Geometry: final body of the model. Coordinates: model frame, mm. A direction names the side the tool comes from. Give positions to 0.01 mm unless a question says otherwise; leave off trailing zeros. Order: outer loops, then holes, each group sorted by start corner. A loop starts at its lowest first (then second) coordinate and runs counter-clockwise, first axis right, second up. Notation, with made-up numbers: (22, -29.5) - (72, -29.5) arc R20 cw to (72, -16.5) - close; hole circle Ø9 at (30, -19). An arc over 180 degrees is marked (long way). Write item = value, one per line. Start each with the question number.
from build123d import *

# Parameters (mm, degrees)
FILLET1_R = 0.5


with BuildPart() as part:
    # Sketch1 → Revolve1 (revolve)
    with BuildSketch(Plane.XY, mode=Mode.PRIVATE) as revolve1_sk:
        Polygon((-80.816688046, 15.015), (-37.316688046, 15.015), (-24.316688046, 15.015), (-24.316688046, 17.5), (27.280476237, 17.5), (54.816688046, 17.5), (54.816688046, 22.5), (59.816688046, 22.5), (59.816688046, 17.5175), (80.816688046, 17.5175), (80.816688046, 0), (-80.816688046, 0), align=None)
    revolve(revolve1_sk.sketch.rotate(Axis((-91.454349808, 0, 0), (1, 0, 0)), 180), axis=Axis((-91.454349808, 0, 0), (1, 0, 0)))

    # Fillet1
    fillet1_edges = [part.edges().sort_by_distance(p)[0] for p in [
        (-24.316688046, 15.015, 0),
        (54.816688046, 17.5, 0),
        (59.816688046, 17.5175, 0),
    ]]
    fillet(fillet1_edges, radius=FILLET1_R)


solid = part.part
Q1. Contact query for flat-ended pins moving along their axis: pin 1 (1 mm diameter, centred on x = 38.5, y = 7.5, fed in from +Z); pin 2 (1.5 mm diameter, centred on x = 10.5, z = -4, fed in from -Y); pin 3 (12 mm diameter, centred on x = -9.5, z = 17.5, fed in from -Y). Output: stop coordinate, or through.
Q2. Section A-A, the plane y = 0. Return the cut outline in (x, z) (1 decimal).
Q3. Material intervals for line 1 along Y through (x, z) = (25, -9); line 2 along Z through (x, y) = (-10.5, 1); line 3 along X through (y, z) = (7, -16.5), sorted ascending. Write a range as from..to.
Q4. Section D-D, the plane x = -14.5. Return the cut outline in (y, z).
Q5. Section C-C, the plane x = -63. Return the cut outline in (y, z) (3 decimals), then the cut area to 3 significant figures.
Q6. Set-up query: faces 1 (the cylindrical face through (57.352, -10.382, 19.961)), 2 (the cylindrical face through (70.71, -16.71, -5.26)), 3 (the flat face through (54.817, -10.1, -15.1)). Return all of +Z, -Z, +X, -X, +Y, -Y with unobstructed straight access to the full face (end or side cutting, diameter ignored); none if empty.
The answers:
q1.pin_1 = 16.04
q1.pin_2 = -17.2
q1.pin_3 = -13.19
q2.outline = (-80.8, -15) - (-24.8, -15) arc R0.5 cw to (-24.3, -15.5) - (-24.3, -17.5) - (54.3, -17.5) arc R0.5 cw to (54.8, -18) - (54.8, -22.5) - (59.8, -22.5) - (59.8, -18) arc R0.5 cw to (60.3, -17.5) - (80.8, -17.5) - (80.8, 17.5) - (60.3, 17.5) arc R0.5 cw to (59.8, 18) - (59.8, 22.5) - (54.8, 22.5) - (54.8, 18) arc R0.5 cw to (54.3, 17.5) - (-24.3, 17.5) - (-24.3, 15.5) arc R0.5 cw to (-24.8, 15) - (-80.8, 15) - close
q3.line_1 = -15.01..15.01
q3.line_2 = -17.47..17.47
q3.line_3 = 54.81..59.83
q4.outline = circle Ø35 at (0, 0)
q5.outline = circle Ø30.03 at (0, 0)
q5.area = 708 mm²
q6.face_1 = +X, -X
q6.face_2 = +X
q6.face_3 = -X
